Can you work these out from the drawing? Everything is in mm from the part's minimum corner. A direction names the side the tool comes from. Coordinates: 2 decimals unless noted, no trailing zeros. Order: outer loops, then holes, each group sorted by start corner. A loop starts at its lowest first (then second) coordinate and runs counter-clockwise, first axis right, second up. Notation, with made-up numbers: M 52,-2.75 L 94,-2.75 A21 cw 94,36.25 Z; hole C 25,0 d5. An arc over 180 degrees is marked long. Answer as CSV lines item,"result". Start each with the question number.
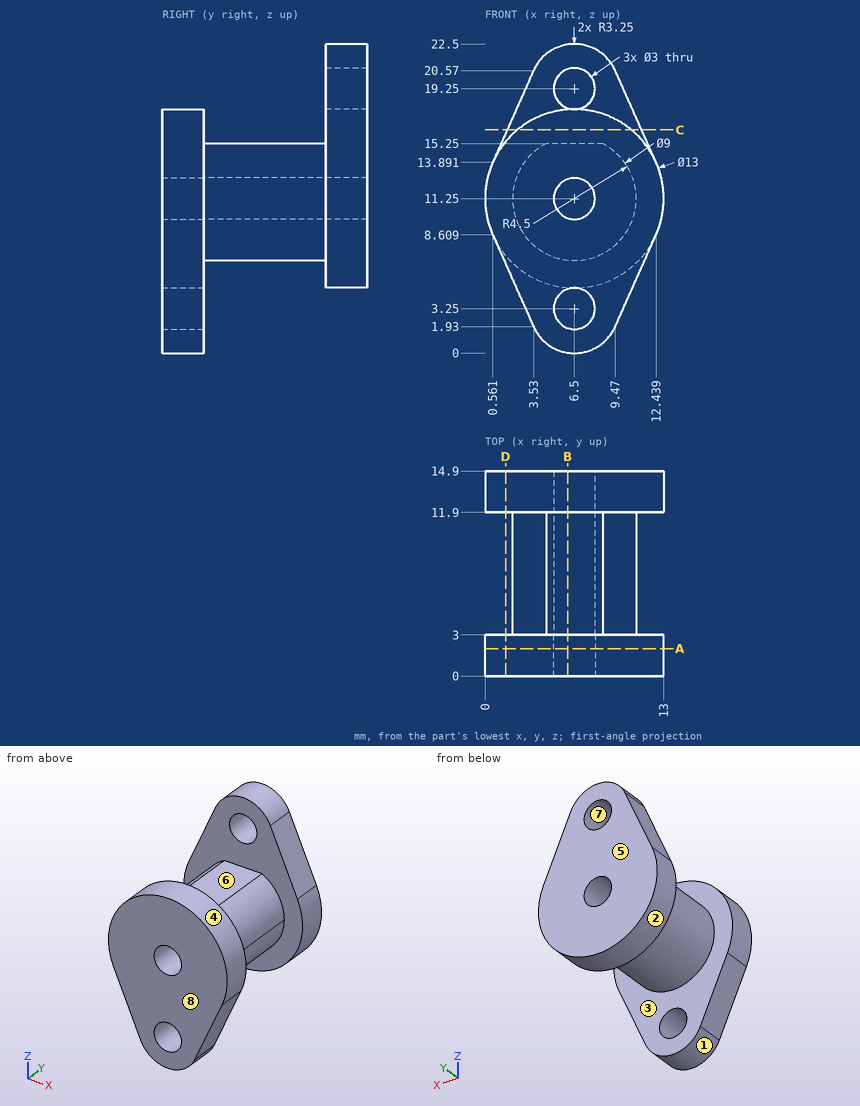
1) Will these pins go through, and if not, where does the flat tip stop? pin 1 Ø2.5 at (x, z) = (6.5, 11.25) entering from -Y; pin 2 Ø1 at (x, y) = (3.5, 12) entering from -Z; pin 3 Ø2 at (x, y) = (8.5, 7.5) entering from +Z; pin 4 Ø4 at (x, y) = (4.5, 4) entering from -Z.
2) I need wall thicknesses on line 1 (Z direction, x = 6.5, y = 1.3); line 2 (Y direction, x = 1.75, z = 12.75); line 3 (Z direction, x = 5.5, y = 13.5) (1 decimal). Which ranges of each line are inside material? Lowest first, please. Write a range as [from, to].
3) Suppose I cut it at D-D on x = 1.5. Please give me the cut outline in (y, z).
4) Suppose I cut it at A-A on y = 2. Please give me the cut outline in (x, z), plus the area to 3 significant figures.
5) Suppose I cut it at C-C on z = 16.25. Please give me the cut outline in (x, y).
6) Which directions (+Z, -Z, +X, -X, +Y, -Y) give clear straight access to the entire face, cutting with the end or side of a thin tool? Please do the marked faces 1, 2, 3, 4 and 5.
7) If we mould it in two halves opening along Y, with no side actions, what happens to the marked faces 6, 7 and 8? For each: released by +Y, released by -Y, zero draft, split by the parting line, or undercut.
8) Suppose I cut it at B-B on x = 6. Give the number of separate pieces and of enclosed holes in the cut face.
Output:
1,pin 1,"through"
1,pin 2,"z = 5.25"
1,pin 3,"z = 15.25"
1,pin 4,"z = 0.01"
2,line 1,"[0, 1.75], [4.75, 9.75], [12.75, 17.75]"
2,line 2,"[0, 3], [11.9, 14.9]"
2,line 3,"[4.8, 10.1], [12.4, 18.1], [20.4, 22.3]"
3,outline,"M 0,6.5 L 3,6.5 L 3,15.4 L 0,15.4 Z; M 11.9,7.1 L 14.9,7.1 L 14.9,16 L 11.9,16 Z"
4,outline,"M 0.56,8.61 L 3.53,1.93 A3.25 ccw 9.47,1.93 L 12.44,8.61 A6.5 ccw long Z; hole C 6.5,3.25 d3; hole C 6.5,11.25 d3"
4,area,"153 mm²"
5,outline,"M 1.61,11.9 L 11.39,11.9 L 11.39,14.9 L 1.61,14.9 Z; M 2.35,0 L 10.65,0 L 10.65,3 L 2.35,3 Z"
6,face 1,"-Z, +Y, -Y"
6,face 2,"+Y"
6,face 3,"none"
6,face 4,"-Y"
6,face 5,"+Z, -Z, +X, -X, +Y"
7,face 6,"undercut"
7,face 7,"zero draft"
7,face 8,"released by -Y"
8,separate pieces,"4"
8,enclosed holes,"0"
